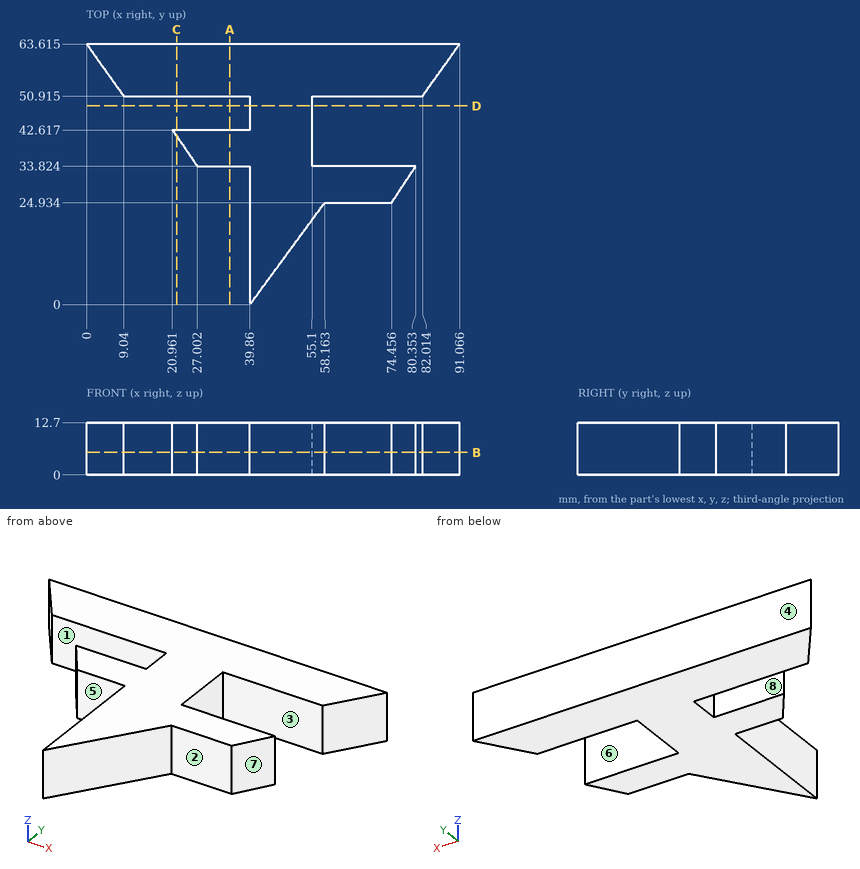
Answer from the drawing. Dimensions are ordinates in mm from the lowest x, y and z of the part. A direction names the side the tool comes from. Coordinates: 2 decimals unless noted, no trailing zeros. Loops run counter-clockwise (first coordinate to the right, second up) from the corner with the lowest first, then second, coordinate; pieces in that order, holes last. Notation, with made-up numbers: (32.25, 2) -> (41.25, 2) arc R23 ccw to (41.25, 28) -> close; hole circle Ø4 at (54, 54). An arc over 180 degrees is marked (long way). Answer in a Markdown table with one row per item.
Item 1: A cutting plane is placed at D-D on y = 48.5. Determine the outline of the cut face in (x, z).
Returned:
| item | result |
|---|---|
| outline | (39.86, 0) -> (55.1, 0) -> (55.1, 12.7) -> (39.86, 12.7) -> close |
Item 2: Straight lines are drawn through the part: line 1 along Y through (x, z) = (33.5, 9.75) (1 decimal); line 2 along Y through (x, z) = (67.5, 6) (1 decimal); line 3 along Y through (x, z) = (11, 10.5) (1 decimal). For each, find the intervals that lie inside material, in ascending order. Write a range as [from, to].
Returned:
| item | result |
|---|---|
| line 1 | y = [33.8, 42.6], [50.9, 63.6] |
| line 2 | y = [24.9, 33.8], [50.9, 63.6] |
| line 3 | y = [50.9, 63.6] |
Item 3: For a pull along Y with two mould halves and no side action, classify the marked faces 1, 2, 3 and 4 as released by +Y, released by -Y, zero draft, split by the parting line, or undercut.
Returned:
| item | result |
|---|---|
| face 1 | undercut |
| face 2 | released by -Y |
| face 3 | undercut |
| face 4 | released by +Y |
Item 4: A cutting plane is placed at B-B on z = 5.5. Determine the outline of the cut face in (x, y) (1 decimal), plus the area to 3 significant figures.
Returned:
| item | result |
|---|---|
| outline | (0, 63.6) -> (9, 50.9) -> (39.9, 50.9) -> (39.9, 42.6) -> (21, 42.6) -> (27, 33.8) -> (39.9, 33.8) -> (39.9, 0) -> (58.2, 24.9) -> (74.5, 24.9) -> (80.4, 33.8) -> (55.1, 33.8) -> (55.1, 50.9) -> (82, 50.9) -> (91.1, 63.6) -> close |
| area | 2,000 mm^2 |
Item 5: For the marked faces 5, 6, 7 and 8, determine the directions among +Z, -Z, +X, -X, +Y, -Y from which every point of the face is accessible in a straight line to the end or side of a thin tool.
Returned:
| item | result |
|---|---|
| face 5 | +Z, -Z, -X, -Y |
| face 6 | +Z, -Z, +X |
| face 7 | +Z, -Z, +X, -Y |
| face 8 | +Z, -Z, -X |
Item 6: A cutting plane is placed at A-A on x = 35. Determine the outline of the cut face in (y, z) (1 decimal), plus the area to 3 significant figures.
Returned:
| item | result |
|---|---|
| outline | (33.8, 0) -> (42.6, 0) -> (42.6, 12.7) -> (33.8, 12.7) -> close; (50.9, 0) -> (63.6, 0) -> (63.6, 12.7) -> (50.9, 12.7) -> close |
| area | 273 mm^2 |
Item 7: A cutting plane is placed at C-C on x = 22. Determine the outline of the cut face in (y, z) (1 decimal).
Returned:
| item | result |
|---|---|
| outline | (41.1, 0) -> (42.6, 0) -> (42.6, 12.7) -> (41.1, 12.7) -> close; (50.9, 0) -> (63.6, 0) -> (63.6, 12.7) -> (50.9, 12.7) -> close |
Item 8: Each of these flat-tipped pins is pushed along its axis until it touches: P1, Ø6.5, axis at x = 67.5, z = 4.5, coming from the -Y side; P2, Ø5, axis at y = 45.5, z = 6, coming from the +X side; P3, Ø2, axis at y = 17, z = 6.5, coming from the +X side. Where does it stop, or does it pass through?
Returned:
| item | result |
|---|---|
| P1 | stops at y = 24.93 |
| P2 | stops at x = 55.1 |
| P3 | stops at x = 53.07 |
